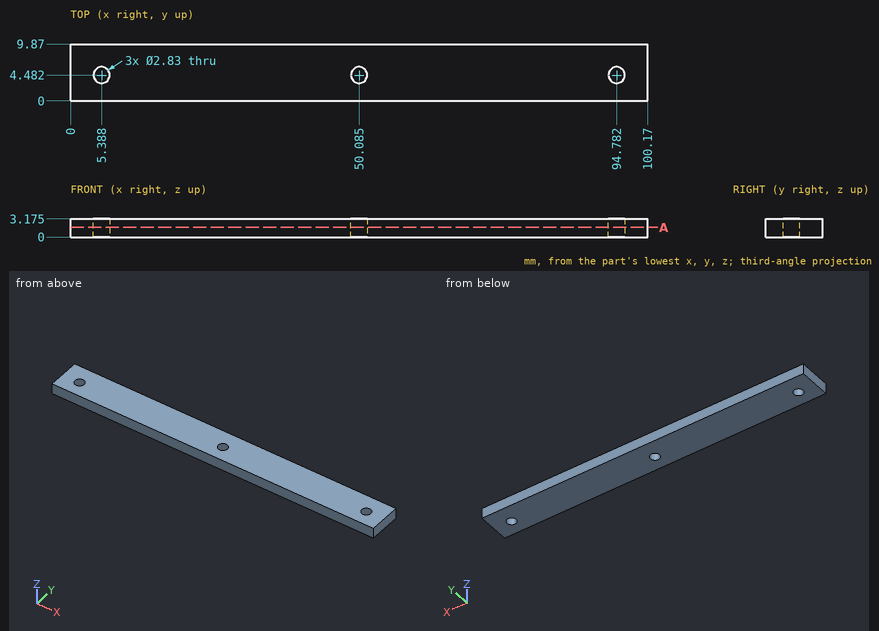
Design review of the part shown in the three views and the two pictorial views. Dimensions are in mm from the part's minimum x, y and z. Round coordinates to 2 decimals unless told otherwise and drop trailing zeros. Order: outer loops, then holes, each group sorted by start corner. A loop starts at its lowest first (then second) coordinate and runs counter-clockwise, first axis right, second up. Notation, with made-up numbers: (81, 78) - (92, 78) arc R9 cw to (92, 90) - close; hole circle Ø5 at (-36, 80.25). An arc over 180 degrees is marked (long way). Answer in a Markdown table with one row per item.
(1) Take a section at A-A on z = 1.7. Write out the cut boundary in (x, y) (1 decimal).
Result set:
| item | result |
|---|---|
| outline | (0, 0) - (100.2, 0) - (100.2, 9.9) - (0, 9.9) - close; hole circle Ø2.8 at (5.4, 4.5); hole circle Ø2.8 at (50.1, 4.5); hole circle Ø2.8 at (94.8, 4.5) |
(2) Clearance check with a flat-ended pin moving along its axis: P1, Ø1.7, axis at x = 5.39, y = 4.48, coming from the -Z side. State where the tip first meets the part, or that it passes through.
Result set:
| item | result |
|---|---|
| P1 | passes through |
(3) For line 1 (X direction, y = 5.75, z = 1.6) (1 decimal); line 2 (X direction, y = 4.75, z = 2.55) (1 decimal); line 3 (Y direction, x = 50.5, z = 0.3) (1 decimal), list the stretches that pass through material, from the lowest coordinate up. Write a range as from..to.
Result set:
| item | result |
|---|---|
| line 1 | x = 0..4.8, 6..49.5, 50.7..94.2, 95.4..100.2 |
| line 2 | x = 0..4, 6.8..48.7, 51.5..93.4, 96.2..100.2 |
| line 3 | y = 0..3.1, 5.8..9.9 |
